Source: CAD feature listing. Evaluate the final solid. Frame: model axes, mm. Face numbers are marked on the shaded views. Give positions to 0.01 mm unless a question says otherwise; leave off trailing zeros. Loops run counter-clockwise (first coordinate to the right, second up) from the corner with the lowest first, then second, coordinate; pieces in that order, holes last.
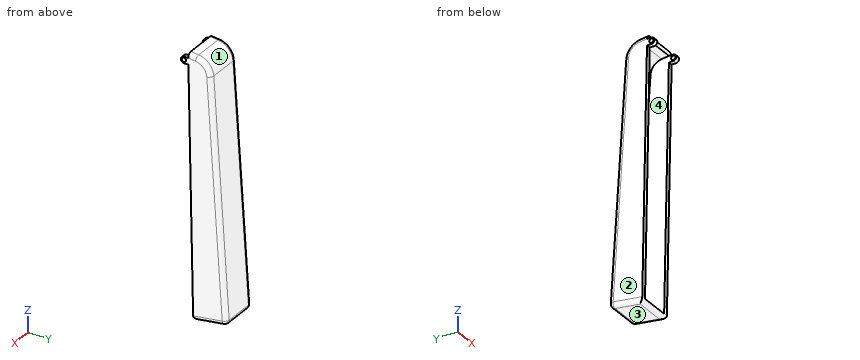
```python
from build123d import *

# Parameters (mm, degrees)
BOSS_EXTRUDE1_DEPTH = 22.86
SHELL3_T            = -2.54
SKETCH2_R           = 1.27
BOSS_EXTRUDE2_DEPTH = 2.54
FILLET2_R           = 2.54


with BuildPart() as part:
    # Sketch1 → Boss-Extrude1 (new body)
    with BuildSketch(Plane(origin=(0, 0, 0), x_dir=(0, 0, -1), z_dir=(1, 0, 0))):
        with BuildLine():
            Line((-95.3996828, -6.597201831), (58.022669589, -3.615128074))
            Line((58.022669589, -3.615128074), (55.274818438, 16.365717982))
            Line((55.274818438, 16.365717982), (-85.421209368, 7.015665501))
            ThreePointArc((-85.421209368, 7.015665501), (-91.73681654, 4.25197608), (-94.834557989, -1.906665904))
            Line((-94.834557989, -1.906665904), (-95.3996828, -6.597201831))
        make_face()
    extrude(amount=BOSS_EXTRUDE1_DEPTH)

    # Shell3
    shell3_openings = [part.faces().sort_by_distance(p)[0] for p in [
        (11.43, -5.106164953, 18.688506605),
    ]]
    offset(amount=SHELL3_T, openings=shell3_openings, kind=Kind.INTERSECTION)

    # Sketch2 → Boss-Extrude2 (add)
    with BuildSketch(Plane(origin=(22.86, 0, 0), x_dir=(0, 0, -1), z_dir=(1, 0, 0))):
        with BuildLine():
            Line((-89.025308756, -6.473302977), (-92.835308756, -6.547358034))
            Line((-92.835308756, -6.547358034), (-92.835308756, -9.087358034))
            ThreePointArc((-92.835308756, -9.087358034), (-90.930308756, -10.992358034), (-89.025308756, -9.087358034))
            Line((-89.025308756, -9.087358034), (-89.025308756, -6.473302977))
        make_face()
        with Locations((-90.930308756, -9.087358034)):
            Circle(SKETCH2_R, mode=Mode.SUBTRACT)
    boss_extrude2 = extrude(amount=-BOSS_EXTRUDE2_DEPTH)

    # Mirror1: Boss-Extrude2 across plane
    add(boss_extrude2.mirror(Plane.ZY.offset(-11.43)))

    # Fillet2
    # the kernel refuses this fillet: 2.54 mm, written as the material it takes off along each edge
    with BuildSketch(Plane(origin=(2.54, 13.674326521, -53.081043163), x_dir=(0, 0.1362419322973002, -0.9906755956840251), z_dir=(-1, 0, 0))) as fillet2_piece_1_section:
        Polygon((0, 0), (FILLET2_R, 0), (FILLET2_R, -FILLET2_R * 0.932051833184), (FILLET2_R * 0.0702509400666, -FILLET2_R * 0.997529350656), align=None)
    fillet2_piece_1 = extrude(amount=FILLET2_R, mode=Mode.PRIVATE)
    fillet2_piece_1 = fillet2_piece_1 - Plane(origin=(2.54, 13.674326521, -53.081043163), x_dir=(0, -0.7751236084755375, 0.6318096165648808), z_dir=(-1, 0, 0)) * Sphere(FILLET2_R, mode=Mode.PRIVATE)
    add(fillet2_piece_1, mode=Mode.SUBTRACT)
    with BuildSketch(Plane(origin=(20.32, 13.674326521, -53.081043163), x_dir=(0, 0.1362419322973002, -0.9906755956840251), z_dir=(1, 0, 0))) as fillet2_piece_2_section:
        Polygon((0, 0), (FILLET2_R, 0), (FILLET2_R, FILLET2_R * 0.932051833184), (FILLET2_R * 0.0702509400666, FILLET2_R * 0.997529350656), align=None)
    fillet2_piece_2 = extrude(amount=FILLET2_R, mode=Mode.PRIVATE)
    fillet2_piece_2 = fillet2_piece_2 - Plane(origin=(20.32, 13.674326521, -53.081043163), x_dir=(0, -0.7751236084755375, 0.6318096165648808), z_dir=(1, 0, 0)) * Sphere(FILLET2_R, mode=Mode.PRIVATE)
    add(fillet2_piece_2, mode=Mode.SUBTRACT)
    with BuildSketch(Plane(origin=(0, -1.906665904, 94.834557989), x_dir=(0, -0.11961688257849476, -0.992820125401476), z_dir=(0, -0.992820125401476, 0.11961688257849475))) as fillet2_piece_3:
        with BuildLine():
            CenterArc((FILLET2_R, FILLET2_R), FILLET2_R, 180, 90)
            Line((0, FILLET2_R), (0, 0))
            Line((0, 0), (FILLET2_R, 0))
        make_face()
    extrude(amount=11.074456935, mode=Mode.SUBTRACT)
    with BuildSketch(Plane(origin=(22.86, -1.906665904, 94.834557989), x_dir=(0, -0.11961688257849476, -0.992820125401476), z_dir=(0, -0.992820125401476, 0.11961688257849475))) as fillet2_piece_4:
        with BuildLine():
            CenterArc((FILLET2_R, -FILLET2_R), FILLET2_R, 90, 90)
            Line((0, -FILLET2_R), (0, 0))
            Line((0, 0), (FILLET2_R, 0))
        make_face()
    extrude(amount=11.074456935, mode=Mode.SUBTRACT)
    with BuildSketch(Plane(origin=(0, -3.121973431, 84.747505515), x_dir=(0, 0.9977991074935991, 0.06630943435874734), z_dir=(0, 0.06630943435874734, -0.9977991074935991))) as fillet2_piece_5:
        with BuildLine():
            CenterArc((10.16 - FILLET2_R, FILLET2_R), FILLET2_R, 270, 90)
            Line((10.16, FILLET2_R), (10.16, 0))
            Line((10.16, 0), (10.16 - FILLET2_R, 0))
        make_face()
    revolve(axis=Axis((0, -3.121973431, 84.747505515), (1, 0, 0)), revolution_arc=79.327967258, mode=Mode.SUBTRACT)
    with BuildSketch(Plane(origin=(22.86, -3.121973431, 84.747505515), x_dir=(0, 0.9977991074935991, 0.06630943435874734), z_dir=(0, 0.06630943435874734, -0.9977991074935991))) as fillet2_piece_6:
        with BuildLine():
            CenterArc((10.16 - FILLET2_R, -FILLET2_R), FILLET2_R, 0, 90)
            Line((10.16, -FILLET2_R), (10.16, 0))
            Line((10.16, 0), (10.16 - FILLET2_R, 0))
        make_face()
    revolve(axis=Axis((22.86, -3.121973431, 84.747505515), (1, 0, 0)), revolution_arc=79.327967258, mode=Mode.SUBTRACT)
    with BuildSketch(Plane(origin=(-7.141741608, -3.615128074, -58.022669589), x_dir=(0, 0.9906755956840251, 0.13624193229729997), z_dir=(1, 0, 0))) as fillet2_piece_7:
        with BuildLine():
            CenterArc((FILLET2_R * 1.12468371782, FILLET2_R), FILLET2_R, 173.283078214, 96.716921786)
            Line((FILLET2_R * 0.131547569233, FILLET2_R * 1.11696405589), (0, 0))
            Line((0, 0), (FILLET2_R * 1.12468371782, 0))
        make_face()
    extrude(amount=37.143483216, mode=Mode.SUBTRACT)
    with BuildSketch(Plane(origin=(0, -9.905918107, -58.887805859), x_dir=(1, 0, 0), z_dir=(0, 0.9906755956840251, 0.1362419322973002))) as fillet2_piece_8:
        with BuildLine():
            CenterArc((FILLET2_R, -FILLET2_R), FILLET2_R, 90, 90)
            Line((0, -FILLET2_R), (0, 0))
            Line((0, 0), (FILLET2_R, 0))
        make_face()
    extrude(amount=24.151497464, mode=Mode.SUBTRACT)
    with BuildSketch(Plane(origin=(22.86, -9.905918107, -58.887805859), x_dir=(-1, 0, 0), z_dir=(0, 0.9906755956840251, 0.1362419322973002))) as fillet2_piece_9:
        with BuildLine():
            CenterArc((FILLET2_R, FILLET2_R), FILLET2_R, 180, 90)
            Line((0, FILLET2_R), (0, 0))
            Line((0, 0), (FILLET2_R, 0))
        make_face()
    extrude(amount=24.151497464, mode=Mode.SUBTRACT)
    with BuildSketch(Plane(origin=(2.54, 16.365717982, -55.274818438), x_dir=(0, -0.9906755956840249, -0.13624193229730105), z_dir=(1, 0, 0))) as fillet2_piece_10:
        with BuildLine():
            CenterArc((FILLET2_R * 0.932051833184, -FILLET2_R), FILLET2_R, 90, 85.971599492)
            Line((-FILLET2_R * 0.065477517472, -FILLET2_R * 0.929749059933), (0, 0))
            Line((0, 0), (FILLET2_R * 0.932051833184, 0))
        make_face()
    extrude(amount=17.78, mode=Mode.SUBTRACT)
    with BuildSketch(Plane(origin=(0, 16.208736254, -52.9126172), x_dir=(1, 0, 0), z_dir=(0, -0.06630943435875185, 0.9977991074935989))) as fillet2_piece_11:
        with BuildLine():
            CenterArc((FILLET2_R, -FILLET2_R), FILLET2_R, 90, 90)
            Line((0, -FILLET2_R), (0, 0))
            Line((0, 0), (FILLET2_R, 0))
        make_face()
    extrude(amount=138.638956008, mode=Mode.SUBTRACT)
    with BuildSketch(Plane(origin=(22.86, 16.208736254, -52.9126172), x_dir=(-1, 0, 0), z_dir=(0, -0.06630943435875185, 0.9977991074935989))) as fillet2_piece_12:
        with BuildLine():
            CenterArc((FILLET2_R, FILLET2_R), FILLET2_R, 180, 90)
            Line((0, FILLET2_R), (0, 0))
            Line((0, 0), (FILLET2_R, 0))
        make_face()
    extrude(amount=138.638956008, mode=Mode.SUBTRACT)


solid = part.part
```
(1) Mould query, pull axis Z, two halves, no side actions, for the marked faces 1, 2, 3 and 4. Classes: pulls with the +Z half, pulls with the -Z half, needs draft (parallel to the pull), parting line crosses it, or undercut.
A:
face 1: pulls with the +Z half
face 2: needs draft
face 3: pulls with the -Z half
face 4: undercut
(2) First-contact query: pin 1 (5 mm diameter, centred on x = 17.5, z = -29.5, fed in from +Y); pin 2 (3 mm diameter, centred on x = 22, y = -7.5, fed in from +Z); pin 3 (1.5 mm diameter, centred on y = -9.09, z = 90.93, fed in from +X); pin 4 (1 mm diameter, centred on x = 19, y = -5, fed in from +Z). Flat tips, straight axial feed; report the tip coordinate or a pass-through.
A:
pin 1: stops at y = 14.82
pin 2: stops at z = 95.35
pin 3: passes through
pin 4: stops at z = 95.27
(3) Section A-A, the plane x = 4.5. Return the cut outline in (y, z).
A:
outline: (-6.6, 95.4) - (-6.55, 92.84) - (-2.21, 92.31) arc R7.62 cw to (4.48, 85.25) - (13.67, -53.08) - (-3.65, -55.46) arc R2.54 ccw to (-0.79, -57.63) - (14.02, -55.6) arc R2.54 ccw to (16.21, -52.91) - (7.02, 85.42) arc R10.16 ccw to (-1.91, 94.83) - close
(4) Ray query, line 1 along X through (y, z) = (7.25, -21.5); line 2 along Y through (x, z) = (4.25, 85.5); line 3 along Z through (x, y) = (20, 3.5). Return the intervals inside material, ascending.
A:
line 1: x = 0 to 2.54, 20.32 to 22.86
line 2: y = 4.46 to 7.01
line 3: z = -57.04 to -54.48, 88.52 to 92.45
